The drawing under review shows one solid part. Ordinate dimensions are in mm from its lowest x, y, z. A direction names the side the tool comes from. Coordinates: 2 decimals unless noted, no trailing zeros. Write each loop counter-clockwise with the first axis right and the second up, starting at its lowest first coordinate (ties: lowest second). Pieces come first, ordered by that corner, then holes. Notation, with made-up numbers: (85.5, -11) - (127.5, -11) arc R15 cw to (127.5, 16) - close; hole circle Ø5 at (55.5, -2). An arc over 180 degrees is marked (long way). Use a Markdown table: item, result.
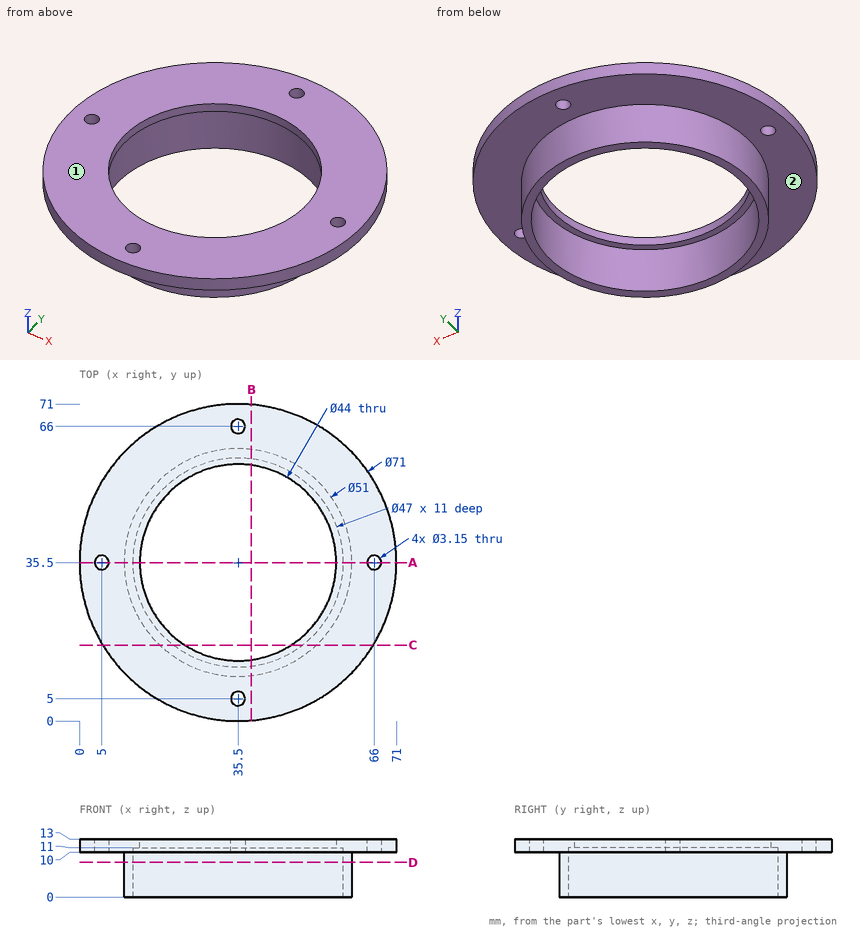
(1) Take a section at B-B on x = 38.5. Write out the cut boundary in (y, z), and give its area (3 significant figures).
Determined:
| item | result |
|---|---|
| outline | (0.13, 10) - (10.18, 10) - (10.18, 0) - (12.19, 0) - (12.19, 11) - (13.71, 11) - (13.71, 13) - (0.13, 13) - close; (57.29, 11) - (58.81, 11) - (58.81, 0) - (60.82, 0) - (60.82, 10) - (70.87, 10) - (70.87, 13) - (57.29, 13) - close |
| area | 119 mm2 |
(2) For L1, parallel to Y at x = 35.5, z = 11.85 (3 decimals); L2, parallel to Y at x = 35.5, z = 7; L3, parallel to Y at x = 35.5, z = 10.7 (3 decimals), list the stretches that pass through material, from the lowest coordinate up. Write a range as from..to.
Determined:
| item | result |
|---|---|
| L1 | 0..3.425, 6.575..13.5, 57.5..64.425, 67.575..71 |
| L2 | 10..12, 59..61 |
| L3 | 0..3.425, 6.575..12, 59..64.425, 67.575..71 |
(3) For pin 1 (1.5 mm diameter, centred on y = 41.5, z = 8, fed in from -X); pin 2 (3.5 mm diameter, centred on x = 35.5, y = 5, fed in from -Z); pin 3 (6 mm diameter, centred on y = 29.5, z = 2, fed in from +X); pin 4 (3 mm diameter, centred on x = 10.5, y = 26.5, fed in from -Z), all flat-tipped, find the tip position at first contact; note any pin that passes through.
Determined:
| item | result |
|---|---|
| pin 1 | x = 10.55 |
| pin 2 | z = 10 |
| pin 3 | x = 60.82 |
| pin 4 | z = 0 |
(4) Take a section at D-D on z = 7.75. Write out the cut boundary in (x, y), and give its area (3 significant figures).
Determined:
| item | result |
|---|---|
| outline | circle Ø51 at (35.5, 35.5); hole circle Ø47 at (35.5, 35.5) |
| area | 308 mm2 |
(5) Take a section at A-A on y = 35.5. Write out the cut boundary in (x, z) (3 decimals), and give its area (3 significant figures).
Determined:
| item | result |
|---|---|
| outline | (0, 10) - (3.425, 10) - (3.425, 13) - (0, 13) - close; (6.575, 10) - (10, 10) - (10, 0) - (12, 0) - (12, 11) - (13.5, 11) - (13.5, 13) - (6.575, 13) - close; (57.5, 11) - (59, 11) - (59, 0) - (61, 0) - (61, 10) - (64.425, 10) - (64.425, 13) - (57.5, 13) - close; (67.575, 10) - (71, 10) - (71, 13) - (67.575, 13) - close |
| area | 99.1 mm2 |
(6) Take a section at C-C on y = 17. Write out the cut boundary in (x, z), and give its area (3 significant figures).
Determined:
| item | result |
|---|---|
| outline | (5.2, 10) - (17.95, 10) - (17.95, 0) - (21.01, 0) - (21.01, 11) - (23.59, 11) - (23.59, 13) - (5.2, 13) - close; (47.41, 11) - (49.99, 11) - (49.99, 0) - (53.05, 0) - (53.05, 10) - (65.8, 10) - (65.8, 13) - (47.41, 13) - close |
| area | 166 mm2 |
(7) Machinability: for the marked faces 1 and 2, which of the approach directions +Z, -Z, +X, -X, +Y, -Y give a long, thin tool a straight path to every point of the face, cutting with its end or side? Answer none if there is none.
Determined:
| item | result |
|---|---|
| face 1 | +Z, +X, -X, +Y, -Y |
| face 2 | -Z |
